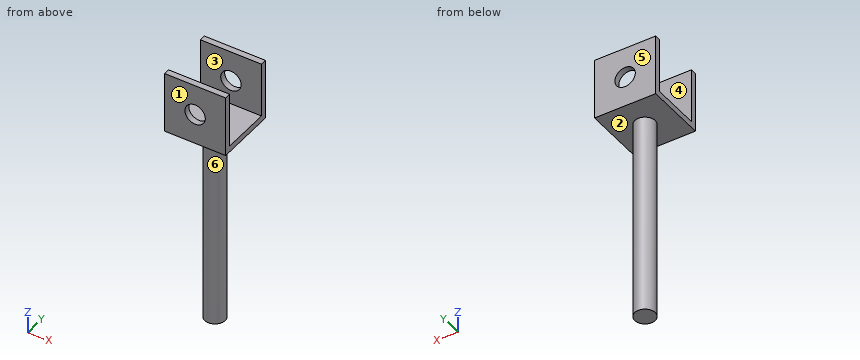
Autodesk Inventor part; units mm, degrees
ref_plane "YZ Plane" through (0, 0, 0) normal (1, 0, 0) x (0, 1, 0)
ref_plane "XZ Plane" through (0, 0, 0) normal (0, 1, 0) x (-1, 0, 0)
ref_plane "XY Plane" through (0, 0, 0) normal (0, 0, 1) x (1, 0, 0)
sketch "Sketch1" plane through (0, 0, 0) normal (1, 0, 0) x (0, 1, 0)
  line L0 (12, 1.5) -> (-12, 1.5)
  line L1 (-15, 1.5) -> (-15, -1.5)
  line L2 (-15, -1.5) -> (15, -1.5)
  line L3 (15, -1.5) -> (15, 1.5)
  line L4 (15, 1.5) -> (-15, -1.5) construction
  line L5 (-15, 1.5) -> (15, -1.5) construction
  line L6 (15, -1.5) -> (12, -1.5)
  line L7 (12, 28.5) -> (15, 28.5)
  line L8 (15, 28.5) -> (15, -1.5)
  line L9 (-15, -1.5) -> (-12, -1.5)
  line L10 (-12, 28.5) -> (-15, 28.5)
  line L11 (-15, 28.5) -> (-15, -1.5)
  line L12 (12, -1.5) -> (12, -1.2)
  line L13 (12, 1.2) -> (12, 28.5)
  line L14 (-12, -1.5) -> (-12, -1.2)
  line L15 (-12, 1.2) -> (-12, 28.5)
  point P0 (0, 0)
  dimension "d0" = 30
  dimension "d1" = 3
  dimension "d2" = 3
  dimension "d3" = 30
  dimension "d4" = 3
  dimension "d5" = 30
extrude "Extrusion1" add sketch "Sketch1" along normal blind 30
sketch "Sketch2" plane through (0, 15, 28.5) normal (0, 1, 0) x (1, 0, 0)
  line L0 (0, 30) -> (30, 30) construction
  line L1 (0, 0) -> (30, 30) construction
  circle A0 centre (15, 15) radius 5
  point P0 (0, 28.5)
  dimension "d8" = 10
extrude "Extrusion2" cut sketch "Sketch2" against normal blind 30
sketch "Sketch3" plane through (0, -15, -1.5) normal (0, 0, -1) x (-1, 0, 0)
  line L0 (0, 0) -> (-30, 0) construction
  line L1 (0, 30) -> (-30, 30) construction
  line L2 (-30, 0) -> (0, 30) construction
  circle A0 centre (-15, 15) radius 5
  point P0 (0, 15)
  dimension "d11" = 10
extrude "Extrusion3" add sketch "Sketch3" along normal blind 100
properties part number "Tensioner"
Geometry: final body of the model. Coordinates: model frame, mm. Face numbers are marked on the shaded views. A direction names the side the tool comes from. Round coordinates to 2 decimals unless told otherwise and drop trailing zeros. Order: outer loops, then holes, each group sorted by start corner. A loop starts at its lowest first (then second) coordinate and runs counter-clockwise, first axis right, second up.
Q1. Section A-A, the plane x = 15. Output: boundary loops of the cut face in (y, z), and give its area (3 significant figures).
Result sheet:
outline: (-15, -1.5) - (-5, -1.5) - (-5, -101.5) - (5, -101.5) - (5, -1.5) - (15, -1.5) - (15, 8.5) - (12, 8.5) - (12, 1.5) - (-12, 1.5) - (-12, 8.5) - (-15, 8.5) - close; (-15, 18.5) - (-12, 18.5) - (-12, 28.5) - (-15, 28.5) - close; (12, 18.5) - (15, 18.5) - (15, 28.5) - (12, 28.5) - close
area: 1,190 mm2
Q2. Section D-D, the plane x = 23.75. Output: boundary loops of the cut face in (y, z).
Result sheet:
outline: (-15, -1.5) - (15, -1.5) - (15, 28.5) - (12, 28.5) - (12, 1.5) - (-12, 1.5) - (-12, 28.5) - (-15, 28.5) - close
Q3. Section C-C, the plane y = 0. Output: boundary loops of the cut face in (x, z), and give its area (3 significant figures).
Result sheet:
outline: (0, -1.5) - (10, -1.5) - (10, -101.5) - (20, -101.5) - (20, -1.5) - (30, -1.5) - (30, 1.5) - (0, 1.5) - close
area: 1,090 mm2
Q4. Access query for the marked faces 4, 5 and 6. Directions: +Z, -Z, +X, -X, +Y, -Y. A direction counts if a zero-diameter tool reaches every point of the face in a straight line with its end or side. Return the directions, or none.
Result sheet:
face 4: +Z, +X, -X
face 5: +Z, -Z, +X, -X, +Y
face 6: -Z
Q5. Section B-B, the plane z = 20.5. Output: boundary loops of the cut face in (x, y), and give its area (3 significant figures).
Result sheet:
outline: (0, -15) - (30, -15) - (30, -12) - (0, -12) - close; (0, 12) - (30, 12) - (30, 15) - (0, 15) - close
area: 180 mm2
Q6. Material intervals for probe 1 along X at (y, z) = (13.8, 13.5); probe 2 along Z at (x, y) = (15, 13.35); probe 3 along Z at (x, y) = (23.75, 8.75), sorted ascending.
Result sheet:
probe 1: x = 0 to 10, 20 to 30
probe 2: z = -1.5 to 8.5, 18.5 to 28.5
probe 3: z = -1.5 to 1.5
Q7. Pin query (flat end, axial travel): pin 1 (8 mm diameter, centred on y = 3, z = -19.5, fed in from -X); pin 2 (3 mm diameter, centred on x = 13, z = -16, fed in from -Y); pin 3 (1.5 mm diameter, centred on x = 19.5, z = -30, fed in from +Y). Return the tip coordinate at first contact, or that it passes through.
Result sheet:
pin 1: stops at x = 10
pin 2: stops at y = -4.97
pin 3: stops at y = 3.31
Q8. Mould query, pull axis Y, two halves, no side actions, for the marked faces 1, 2 and 3. Classes: released by +Y, released by -Y, zero draft, split by the parting line, or undercut.
Result sheet:
face 1: released by -Y
face 2: zero draft
face 3: undercut
